Read the model definition and answer for the solid it produces. Units are mm, in the model's axes. Face numbers are marked on the shaded views. A direction names the side the tool comes from. Coordinates: 2 decimals unless noted, no trailing zeros. Loops run counter-clockwise (first coordinate to the right, second up) from the corner with the lowest first, then second, coordinate; pieces in that order, holes last.
from build123d import *

# Parameters (mm, degrees)
F0_W      = 64
F0_H      = 18
F1_DEPTH  = 48
F2_W      = 64
F2_H      = 1
F3_DEPTH  = 32
F4_W      = 30.5
F4_H      = 15
F5_DEPTH  = 15
F6_W      = 32
F6_H      = 46
F7_DEPTH  = 1
F9_DEPTH  = 1
F11_DEPTH = 1


with BuildPart() as f1:
    # F0 (on Top) → F1 (new body)
    with BuildSketch(Plane.XY):
        with Locations((32, 9)):
            Rectangle(F0_W, F0_H)
    extrude(amount=F1_DEPTH)

    # F2 (on face) → F3 (join)
    with BuildSketch(Plane.XY.offset(48)):
        with Locations((32, 17.5)):
            Rectangle(F2_W, F2_H)
    extrude(amount=F3_DEPTH)

    # F4 (on face) → F5 (join)
    with BuildSketch(Plane.XZ.offset(-17)):
        Polygon((1, 80), (0, 80), (0, 79), (0, 64), (0, 63), (0, 48), (1, 48), (1, 63), (31.5, 63), (31.5, 48), (32.5, 48), (32.5, 63), (63, 63), (63, 48), (64, 48), (64, 79), (64, 80), (63, 80), (32.5, 80), (31.5, 80), align=None)
        with Locations((16.25, 71.5)):
            Rectangle(F4_W, F4_H, mode=Mode.SUBTRACT)
        with Locations((47.75, 71.5)):
            Rectangle(F4_W, F4_H, mode=Mode.SUBTRACT)
    extrude(amount=F5_DEPTH)

    # F6 (on face) → F7 (cut)
    with BuildSketch(Plane.XZ):
        with Locations((48, 24)):
            Rectangle(F6_W, F6_H)
    extrude(amount=-F7_DEPTH, mode=Mode.SUBTRACT)

    # F8 (on face) → F9 (cut)
    with BuildSketch(Plane.XZ.offset(-1)):
        with BuildLine():
            ThreePointArc((63, 42), (61.93934, 41.56066), (61.5, 40.5))
            Line((61.5, 40.5), (61.5, 37.5))
            ThreePointArc((61.5, 37.5), (61.93934, 36.43934), (63, 36))
            Line((63, 36), (63, 42))
        make_face()
    extrude(amount=-F9_DEPTH, mode=Mode.SUBTRACT)

    # F10 (on face) → F11 (cut)
    with BuildSketch(Plane.XZ):
        with BuildLine():
            ThreePointArc((2.5, 40.5), (2.06066, 41.56066), (1, 42))
            Line((1, 42), (1, 36))
            ThreePointArc((1, 36), (2.06066, 36.43934), (2.5, 37.5))
            Line((2.5, 37.5), (2.5, 40.5))
        make_face()
    extrude(amount=-F11_DEPTH, mode=Mode.SUBTRACT)


solid = f1.part
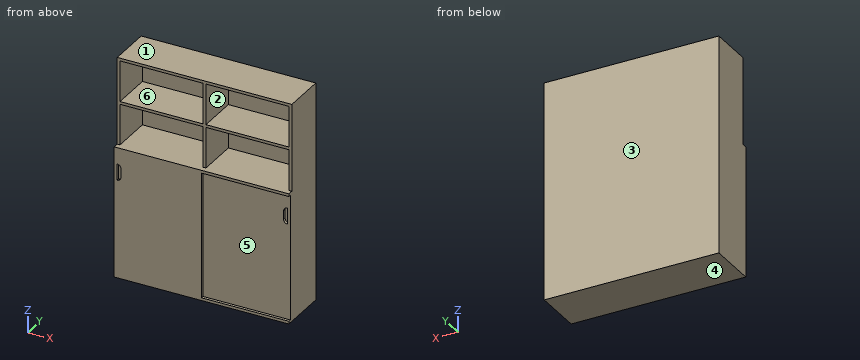
Q1. Which of the six approach directions +Z, -Z, +X, -X, +Y, -Y give full straight-line access (tool end or side, diameter ignored) to the marked faces 4, 5 and 6?
Findings below:
face 4: -Z, +X, -X, +Y, -Y
face 5: +X, -Y
face 6: -Y
Q2. A cutting plane is placed at A-A (y = 9.25). Give the vertices of the cut face in (x, z).
Findings below:
outline: (0, 0) - (64, 0) - (64, 80) - (0, 80) - close; hole (1, 48) - (31.5, 48) - (31.5, 63) - (1, 63) - close; hole (1, 64) - (31.5, 64) - (31.5, 79) - (1, 79) - close; hole (32.5, 48) - (63, 48) - (63, 63) - (32.5, 63) - close; hole (32.5, 64) - (63, 64) - (63, 79) - (32.5, 79) - close
Q3. A cutting plane is placed at C-C (z = 9). Give the vertices of the cut face in (x, y), then the cut area to 3 significant figures.
Findings below:
outline: (0, 0) - (32, 0) - (32, 1) - (64, 1) - (64, 18) - (0, 18) - close
area: 1,120 mm2
Q4. Flat-ended cylindrical pins translate along their axes: pin 1 Ø0.5 at (y, z) = (0.5, 12.5) entering from +X; pin 2 Ø5 at (x, z) = (8, 58) entering from -Y; pin 3 Ø9.5 at (x, z) = (32, 68.5) entering from -Y. Find the tip coordinate at first contact, or state that the pin passes through.
Findings below:
pin 1: stops at x = 32
pin 2: stops at y = 17
pin 3: stops at y = 2
Q5. A cutting plane is placed at D-D (x = 45.5). Give the vertices of the cut face in (y, z).
Findings below:
outline: (0, 0) - (18, 0) - (18, 80) - (2, 80) - (2, 79) - (17, 79) - (17, 64) - (2, 64) - (2, 63) - (17, 63) - (17, 48) - (0, 48) - (0, 47) - (1, 47) - (1, 1) - (0, 1) - close
Q6. Determine the mould class of the marked faces 1, 2 and 3 for opening direction Z: +Z half, -Z half, draft (parallel to the pull), parting line (faces both ways), or undercut.
Findings below:
face 1: +Z half
face 2: undercut
face 3: draft
Q7. A cutting plane is placed at B-B (x = 16.5). Give the vertices of the cut face in (y, z).
Findings below:
outline: (0, 0) - (18, 0) - (18, 80) - (2, 80) - (2, 79) - (17, 79) - (17, 64) - (2, 64) - (2, 63) - (17, 63) - (17, 48) - (0, 48) - close
Q8. Straight lines are drawn through the part: probe 1 along X at (y, z) = (14.5, 54.5); probe 2 along Z at (x, y) = (26, 12.25); probe 3 along Y at (x, z) = (29.5, 52.5). For each, find the intervals that lie inside material, in ascending order.
Findings below:
probe 1: x = 0 to 1, 31.5 to 32.5, 63 to 64
probe 2: z = 0 to 48, 63 to 64, 79 to 80
probe 3: y = 17 to 18
